Here's how the part is built. I have some questions about the finished solid (model axes, mm). Round coordinates to 2 decimals unless told otherwise and drop trailing zeros. Loops run counter-clockwise (first coordinate to the right, second up) from the corner with the lowest first, then second, coordinate; pieces in that order, holes last. Notation, with made-up numbers: M -37.5,-22.5 L -17.5,-22.5 A18 cw -17.5,-0.5 Z; hole C -3,61 d5. An arc over 180 degrees is marked long. Answer as a JSON object with one key per item and string values.
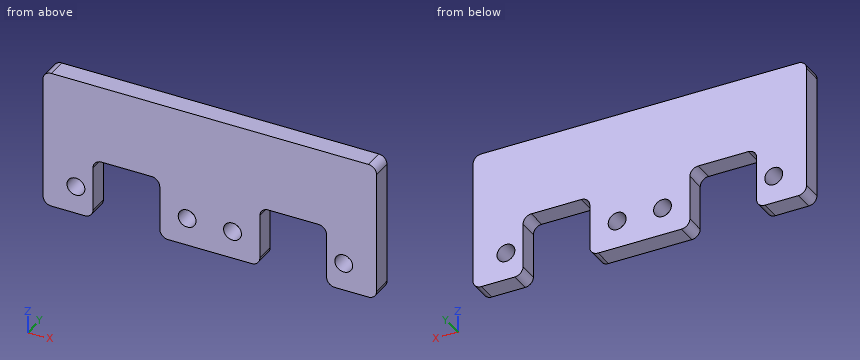
from build123d import *

# Parameters (mm, degrees)
BOSS_EXTRUDE1_DEPTH   = 3.5
F_2_CLEARANCE_HOLE1_D = 3.2131
FILLET1_R             = 1.5


with BuildPart() as part:
    # Sketch1 → Boss-Extrude1 (new body)
    with BuildSketch(Plane(origin=(0, 0, 0), x_dir=(1, 0, 0), z_dir=(0, 1, 0))):
        Polygon((-21, 12.5), (-21, 1.5), (-9, 1.5), (-9, 12.5), (9, 12.5), (9, 1.5), (21, 1.5), (21, 12.5), (30, 12.5), (30, -12.5), (-30, -12.5), (-30, 12.5), align=None)
    extrude(amount=BOSS_EXTRUDE1_DEPTH)

    # #2 Clearance Hole1 (through all)
    with Locations(Plane(origin=(0, 3.5, 0), x_dir=(1, 0, 0), z_dir=(0, 1, 0))):
        with Locations((24.079999968, 7.5), (-24.079999968, 7.5), (-4.079999968, 7.5), (4.079999968, 7.5)):
            Hole(F_2_CLEARANCE_HOLE1_D / 2)

    # Fillet1
    fillet1_edges = [part.edges().sort_by_distance(p)[0] for p in [
        (30, 1.75, -12.5),
        (30, 1.75, 12.5),
        (-30, 1.75, 12.5),
        (-30, 1.75, -12.5),
        (-21, 1.75, -12.5),
        (-21, 1.75, -1.5),
        (-9, 1.75, -1.5),
        (-9, 1.75, -12.5),
        (9, 1.75, -12.5),
        (9, 1.75, -1.5),
        (21, 1.75, -1.5),
        (21, 1.75, -12.5),
    ]]
    fillet(fillet1_edges, radius=FILLET1_R)


solid = part.part
Item 1: I want a section at A-A on x = -4.08. List the corners of the cut face in (y, z) for me, plus the area to 3 significant figures.
Solution:
{"outline": "M 0,-12.5 L 3.5,-12.5 L 3.5,-9.11 L 0,-9.11 Z; M 0,-5.89 L 3.5,-5.89 L 3.5,12.5 L 0,12.5 Z", "area": "76.3 mm2"}
Item 2: If I drill on L1, parallel to X at y = 1.3, z = -3.25; L2, parallel to Z at x = -4, y = 2.5; L3, parallel to Z at x = 5, y = 1.2, over which ranges is the centre line in solid material (lowest first)? Write a range as from..to.
Solution:
{"L1": "x = -30..-21, -9..9, 21..30", "L2": "z = -12.5..-9.1, -5.9..12.5", "L3": "z = -12.5..-8.82, -6.18..12.5"}
Item 3: For P1, Ø1, axis at x = -14.5, y = 1.5, coming from the -Z side, with a flat end and sliding along its axis, tell me the tip position at first contact or that it passes through.
Solution:
{"P1": "stops at z = -1.5"}
Item 4: I want a section at C-C on y = 1.15. List the corners of the cut face in (x, z) for me.
Solution:
{"outline": "M -30,-11 A1.5 ccw -28.5,-12.5 L -22.5,-12.5 A1.5 ccw -21,-11 L -21,-3 A1.5 cw -19.5,-1.5 L -10.5,-1.5 A1.5 cw -9,-3 L -9,-11 A1.5 ccw -7.5,-12.5 L 7.5,-12.5 A1.5 ccw 9,-11 L 9,-3 A1.5 cw 10.5,-1.5 L 19.5,-1.5 A1.5 cw 21,-3 L 21,-11 A1.5 ccw 22.5,-12.5 L 28.5,-12.5 A1.5 ccw 30,-11 L 30,11 A1.5 ccw 28.5,12.5 L -28.5,12.5 A1.5 ccw -30,11 Z; hole C -24.08,-7.5 d3.21; hole C -4.08,-7.5 d3.21; hole C 4.08,-7.5 d3.21; hole C 24.08,-7.5 d3.21"}
Item 5: I want a section at B-B on z = -7.5. List the corners of the cut face in (x, y) for me, plus the area to 3 significant figures.
Solution:
{"outline": "M -30,0 L -25.69,0 L -25.69,3.5 L -30,3.5 Z; M -22.47,0 L -21,0 L -21,3.5 L -22.47,3.5 Z; M -9,0 L -5.69,0 L -5.69,3.5 L -9,3.5 Z; M -2.47,0 L 2.47,0 L 2.47,3.5 L -2.47,3.5 Z; M 5.69,0 L 9,0 L 9,3.5 L 5.69,3.5 Z; M 21,0 L 22.47,0 L 22.47,3.5 L 21,3.5 Z; M 25.69,0 L 30,0 L 30,3.5 L 25.69,3.5 Z", "area": "81.0 mm2"}
Item 6: I want a section at D-D on x = 18. List the corners of the cut face in (y, z) for me.
Solution:
{"outline": "M 0,-1.5 L 3.5,-1.5 L 3.5,12.5 L 0,12.5 Z"}
